```python
from build123d import *

# Parameters (mm, degrees)
SKETCH_R   = 1.2
SKETCH_R_2 = 2
SKETCH_W   = 4
SKETCH_H   = 22
PAD_DEPTH  = 4


with BuildPart() as part:
    # Sketch → Pad (new body)
    with BuildSketch(Plane.XY):
        Polygon((0, 0), (33.5, 0), (33.5, 4), (37.75, 8.25), (41.75, 8.25), (41.75, 41.75), (37.75, 41.75), (33.5, 46), (33.5, 50), (0, 50), (0, 46), (-4.25, 41.75), (-8.25, 41.75), (-8.25, 8.25), (-4.25, 8.25), (0, 4), align=None)
        with Locations((-1.25, 34.75)):
            Circle(SKETCH_R, mode=Mode.SUBTRACT)
        with Locations((-1.25, 14.75)):
            Circle(SKETCH_R, mode=Mode.SUBTRACT)
        with Locations((34.75, 14.75)):
            Circle(SKETCH_R, mode=Mode.SUBTRACT)
        with Locations((34.75, 34.75)):
            Circle(SKETCH_R, mode=Mode.SUBTRACT)
        with Locations((23.75, 32)):
            Circle(SKETCH_R_2, mode=Mode.SUBTRACT)
        with Locations((5.25, 21)):
            Rectangle(SKETCH_W, SKETCH_H, mode=Mode.SUBTRACT)
        with Locations((28.25, 21)):
            Rectangle(SKETCH_W, SKETCH_H, mode=Mode.SUBTRACT)
    extrude(amount=PAD_DEPTH)


solid = part.part
```
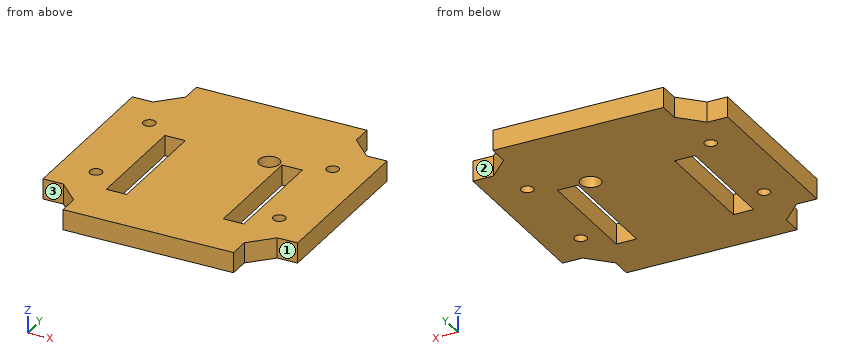
Geometry check sheet. Reference: the model listing, model coordinates, mm. Face numbers are marked on the shaded views. A direction names the side the tool comes from. Give positions to 0.01 mm unless a question says otherwise; leave off trailing zeros. Loops run counter-clockwise (first coordinate to the right, second up) from the corner with the lowest first, then second, coordinate; pieces in that order, holes last. Notation, with made-up numbers: M 66,-7 L 121,-7 A20 ccw 121,17 Z; hole C -25.5,-4 d8. An arc over 180 degrees is marked long. Write item = value, one per line. Start each with the question number.
1. Section check D-D, the plane z = 3.4. Give the number of separate pieces and of enclosed holes in the cut face, plus the area to 3 significant figures.
2. Go/stop test with flat-tipped pins: P1, Ø1.2, axis at x = 40.5, z = 2.5, coming from the -Y side; P2, Ø1.2, axis at y = 1.5, z = 1.5, coming from the +X side; P3, Ø1.2, axis at y = 2.5, z = 2, coming from the -X side. Record where each tip stops, or that it passes through.
3. Section check C-C, the plane x = 23.75. Enter the section's corners in (y, z), plus the area to 3 significant figures.
4. Tool access check on the marked faces 1, 2 and 3. Record the directions out of +Z, -Z, +X, -X, +Y, -Y that give a thin tool (end or side, any length) a straight path to the whole face; none if there is none.
5. Thickness scan on probe 1 along X at (y, z) = (24.5, 3); probe 2 along Y at (x, z) = (34.75, 0.95). Record the ranges inside material, lowest first.
6. Section check A-A, the plane x = -1.25. Enter the section's corners in (y, z), plus the area to 3 significant figures.
7. Section check B-B, the plane y = 34.75. Enter the section's corners in (x, z).
Values follow:
q1.separate_pieces = 1
q1.enclosed_holes = 7
q1.area = 2,060 mm^2
q2.P1 = 8.25
q2.P2 = 33.5
q2.P3 = 0
q3.outline = M 0,0 L 30,0 L 30,4 L 0,4 Z; M 34,0 L 50,0 L 50,4 L 34,4 Z
q3.area = 184 mm^2
q4.face_1 = +Z, -Z, +X, -Y
q4.face_2 = +Z, -Z, +X, +Y
q4.face_3 = +Z, -Z, -X, -Y
q5.probe_1 = -8.25 to 3.25, 7.25 to 26.25, 30.25 to 41.75
q5.probe_2 = 5.25 to 13.55, 15.95 to 33.55, 35.95 to 44.75
q6.outline = M 5.25,0 L 13.55,0 L 13.55,4 L 5.25,4 Z; M 15.95,0 L 33.55,0 L 33.55,4 L 15.95,4 Z; M 35.95,0 L 44.75,0 L 44.75,4 L 35.95,4 Z
q6.area = 139 mm^2
q7.outline = M -8.25,0 L -2.45,0 L -2.45,4 L -8.25,4 Z; M -0.05,0 L 33.55,0 L 33.55,4 L -0.05,4 Z; M 35.95,0 L 41.75,0 L 41.75,4 L 35.95,4 Z
